Answer from the drawing. Dimensions are ordinates in mm from the lowest x, y and z of the part. Give positions to 0.01 mm unless a question says otherwise; leave off trailing zeros. Order: outer loops, then holes, each group sorted by start corner. A loop starts at its lowest first (then second) coordinate and runs counter-clockwise, first axis right, second up. Notation, with made-up numbers: (15.25, 21.25) - (59.25, 21.25) arc R31 cw to (59.25, 45.25) - close; hole circle Ø5 at (84, -27.5). An arc over 180 degrees is marked (long way). Use a Markdown table: item, result. Add a question column.
1) Find section C-C, the plane x = 10.5. Determine the outline of the cut face in (y, z), plus the area to 3 significant figures.
2) Find section A-A, the plane z = 5. Determine the outline of the cut face in (x, y).
3) Straight lines are drawn through the part: line 1 (Y direction, x = 128.5, z = 2); line 2 (X direction, y = 133.5, z = 4.5); line 3 (Y direction, x = 7.5, z = 5.25). For each, find the intervals that lie inside material, in ascending order.
4) Find section B-B, the plane y = 13. Determine the outline of the cut face in (x, z), plus the area to 3 significant figures.
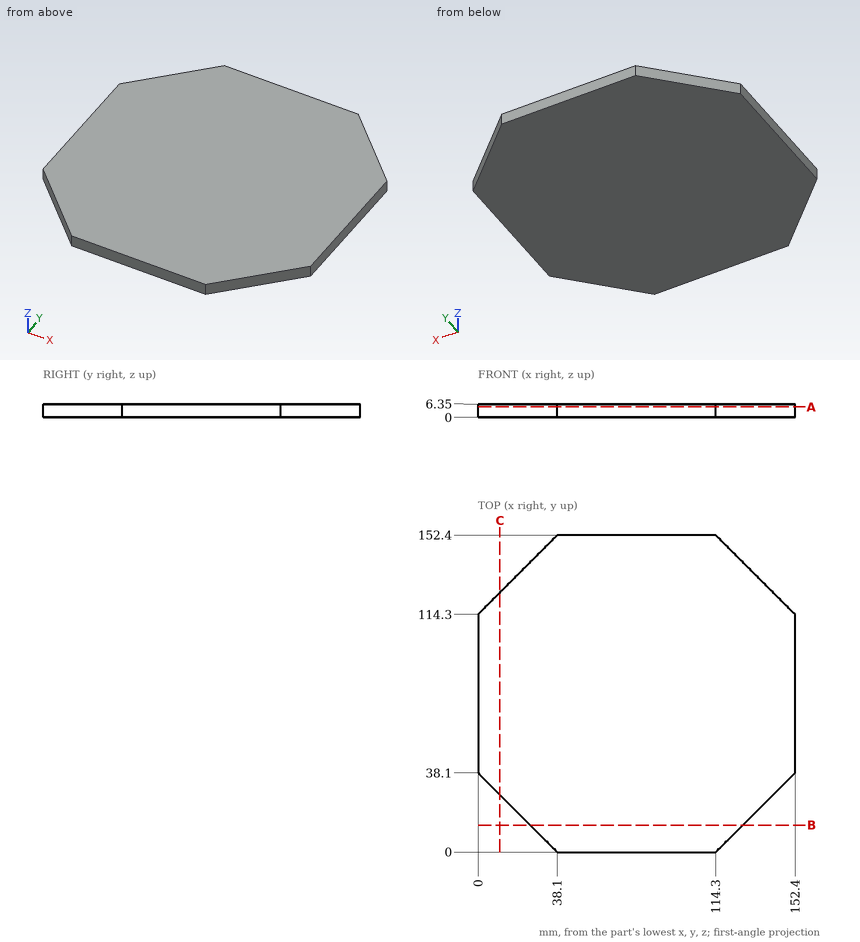
The answers:
| question | item | result |
|---|---|---|
| 1 | outline | (27.6, 0) - (124.8, 0) - (124.8, 6.35) - (27.6, 6.35) - close |
| 1 | area | 617 mm2 |
| 2 | outline | (0, 38.1) - (38.1, 0) - (114.3, 0) - (152.4, 38.1) - (152.4, 114.3) - (114.3, 152.4) - (38.1, 152.4) - (0, 114.3) - close |
| 3 | line 1 | 14.2 to 138.2 |
| 3 | line 2 | 19.2 to 133.2 |
| 3 | line 3 | 30.6 to 121.8 |
| 4 | outline | (25.1, 0) - (127.3, 0) - (127.3, 6.35) - (25.1, 6.35) - close |
| 4 | area | 649 mm2 |
